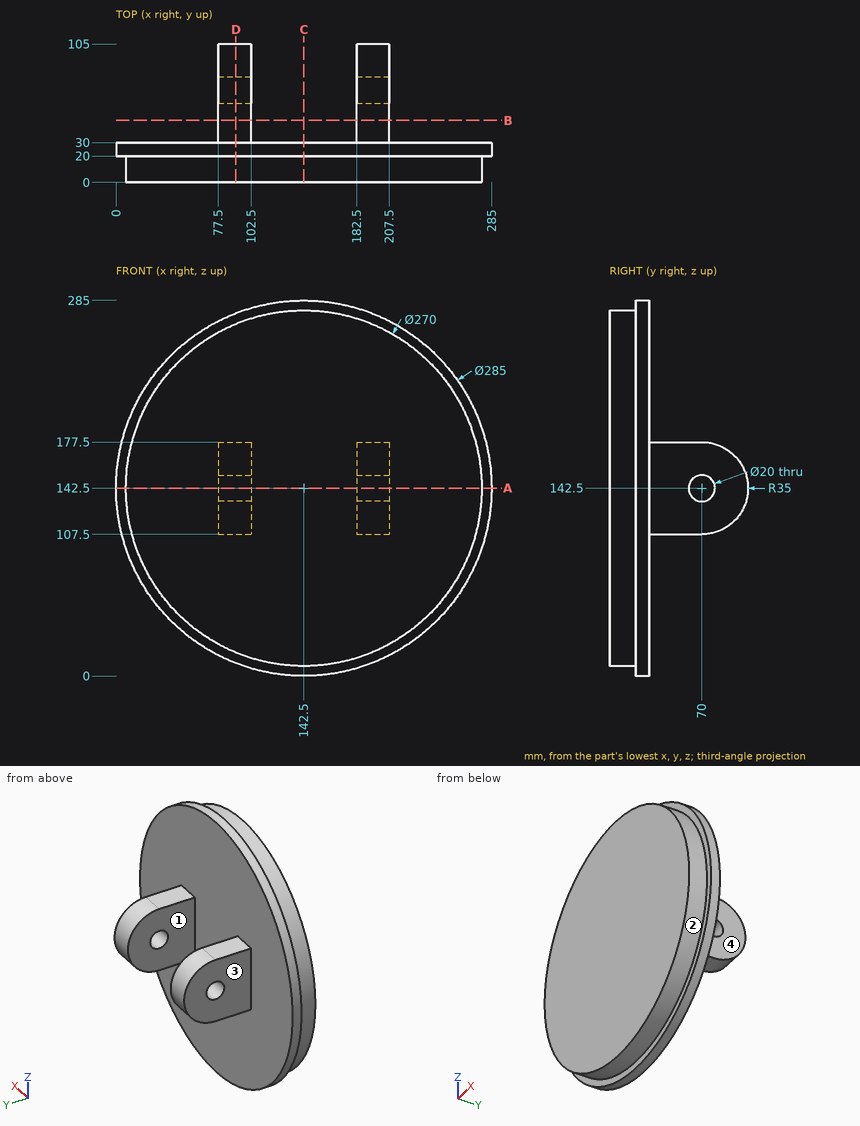
Job drawing, mm, ordinate dimensions from the low corner. One solid piece. A direction names the side the tool comes from. Give positions to 0.01 mm unless a question says otherwise; leave off trailing zeros. Loops run counter-clockwise (first coordinate to the right, second up) from the corner with the lowest first, then second, coordinate; pieces in that order, holes last. Notation, with made-up numbers: M -9.5,-10.5 L 41.5,-10.5 A8 ccw 41.5,-3.5 Z; hole C 66.25,67 d3. An arc over 180 degrees is marked long. Answer in a Markdown table with one row per item. Add a question column.
Item 1: Band-saw the part on C-C on x = 142.5. Give the cut face in (y, z), then the cut area to 3 significant figures.
Item 2: Band-saw the part on B-B on y = 47. Give the cut face in (x, z), then the cut area to 3 significant figures.
Item 3: Band-saw the part on D-D on x = 91. Give the cut face in (y, z), then the cut area to 3 significant figures.
Item 4: Drop flat-ended pins along their axis: P1, Ø20, axis at x = 95.5, y = 48.5, coming from the +Z side; P2, Ø3, axis at y = 84.5, z = 165, coming from the -X side; P3, Ø1, axis at y = 74, z = 119.5, coming from the +X side; P4, Ø5, axis at x = 112, z = 155.5, coming from the -Y side. Give the stop position or say it passes through.
Item 5: Tool access for the marked faces 1, 2, 3 and 4: list every direction of +Z, -Z, +X, -X, +Y, -Y with a clear straight run to the whole face (end or side of a thin tool).
Item 6: Band-saw the part on A-A on z = 142.5. Give the cut face in (x, y), then the cut area to 3 significant figures.
Item 7: Probe probe 1 along Y at (x, z) = (95, 142); probe 2 along X at (y, z) = (90.5, 144); probe 3 along Y at (x, z) = (210.5, 88). List the from-to ranges inside material, lowest first.
Reply:
| question | item | result |
|---|---|---|
| 1 | outline | M 0,7.5 L 20,7.5 L 20,0 L 30,0 L 30,285 L 20,285 L 20,277.5 L 0,277.5 Z |
| 1 | area | 8,250 mm^2 |
| 2 | outline | M 77.5,107.5 L 102.5,107.5 L 102.5,177.5 L 77.5,177.5 Z; M 182.5,107.5 L 207.5,107.5 L 207.5,177.5 L 182.5,177.5 Z |
| 2 | area | 3,500 mm^2 |
| 3 | outline | M 0,17.71 L 20,17.71 L 20,9.63 L 30,9.63 L 30,107.5 L 70,107.5 A35 ccw 70,177.5 L 30,177.5 L 30,275.37 L 20,275.37 L 20,267.29 L 0,267.29 Z; hole C 70,142.5 d20 |
| 3 | area | 12,100 mm^2 |
| 4 | P1 | stops at z = 177.5 |
| 4 | P2 | stops at x = 77.5 |
| 4 | P3 | stops at x = 207.5 |
| 4 | P4 | stops at y = 0 |
| 5 | face 1 | +Z, -Z, +Y |
| 5 | face 2 | -Y |
| 5 | face 3 | +Z, -Z, -X, +Y |
| 5 | face 4 | +Z, -Z, +X, +Y |
| 6 | outline | M 0,20 L 7.5,20 L 7.5,0 L 277.5,0 L 277.5,20 L 285,20 L 285,30 L 207.5,30 L 207.5,60 L 182.5,60 L 182.5,30 L 102.5,30 L 102.5,60 L 77.5,60 L 77.5,30 L 0,30 Z; M 77.5,80 L 102.5,80 L 102.5,105 L 77.5,105 Z; M 182.5,80 L 207.5,80 L 207.5,105 L 182.5,105 Z |
| 6 | area | 11,000 mm^2 |
| 7 | probe 1 | y = 0 to 60.01, 79.99 to 105 |
| 7 | probe 2 | x = 77.5 to 102.5, 182.5 to 207.5 |
| 7 | probe 3 | y = 0 to 30 |
